```python
from build123d import *

# Parameters (mm, degrees)
SKETCH1_R           = 13.85
BOSS_EXTRUDE1_DEPTH = 12.3
SKETCH2_R           = 8.625
BOSS_EXTRUDE2_DEPTH = 1.7
SKETCH3_R           = 4.6
BOSS_EXTRUDE3_DEPTH = 8
SKETCH4_R           = 2.955
BOSS_EXTRUDE4_DEPTH = 11.75
SKETCH5_R           = 1.5
BOSS_EXTRUDE5_DEPTH = 3.42


with BuildPart() as part:
    # Sketch1 → Boss-Extrude1 (new body)
    with BuildSketch(Plane(origin=(0, 0, 0), x_dir=(1, 0, 0), z_dir=(0, 1, 0))):
        with Locations(Location((0, 0, 0), (0, 0, 270))):
            Circle(SKETCH1_R)
    extrude(amount=BOSS_EXTRUDE1_DEPTH)

    # Sketch2 → Boss-Extrude2 (add)
    with BuildSketch(Plane(origin=(0, 12.3, 0), x_dir=(1, 0, 0), z_dir=(0, 1, 0))):
        with Locations(Location((0, 0, 0), (0, 0, 270))):
            Circle(SKETCH2_R)
    extrude(amount=BOSS_EXTRUDE2_DEPTH)

    # Sketch3 → Boss-Extrude3 (add)
    with BuildSketch(Plane(origin=(0, 14, 0), x_dir=(1, 0, 0), z_dir=(0, 1, 0))):
        with Locations(Location((0, 0, 0), (0, 0, 270))):
            Circle(SKETCH3_R)
    extrude(amount=BOSS_EXTRUDE3_DEPTH)

    # Sketch4 → Boss-Extrude4 (add)
    with BuildSketch(Plane(origin=(0, 22, 0), x_dir=(1, 0, 0), z_dir=(0, 1, 0))):
        with Locations(Location((0, 0, 0), (0, 0, 270))):
            Circle(SKETCH4_R)
    extrude(amount=BOSS_EXTRUDE4_DEPTH)

    # Sketch5 → Boss-Extrude5 (add)
    with BuildSketch(Plane(origin=(0, 12.3, 0), x_dir=(1, 0, 0), z_dir=(0, 1, 0))):
        with Locations(Location((0, 9.7, 0), (0, 0, 228.961978667))):
            Circle(SKETCH5_R)
    extrude(amount=BOSS_EXTRUDE5_DEPTH)


solid = part.part
```
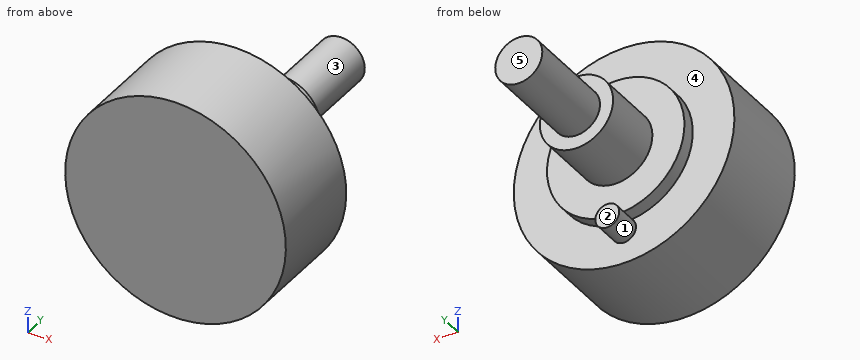
Build history of the part. All positions in model axes, mm. Face numbers are marked on the shaded views. A direction names the side the tool comes from. Give positions to 0.01 mm unless a question says otherwise; leave off trailing zeros. Order: outer loops, then holes, each group sorted by start corner. A loop starts at its lowest first (then second) coordinate and runs counter-clockwise, first axis right, second up. Notation, with made-up numbers: M -22,10 L 37,10 A11 ccw 37,25 Z; hole C -21.5,13.5 d1. An arc over 180 degrees is marked long. Return JSON: item names as keys, results as strings.
Q1. Band-saw the part on B-B (z = 0). Give the cut face in (x, y) (3 decimals), then the cut area to 3 significant figures.
Answer list:
{"outline": "M -13.85,0 L 13.85,0 L 13.85,12.3 L 8.625,12.3 L 8.625,14 L 4.6,14 L 4.6,22 L 2.955,22 L 2.955,33.75 L -2.955,33.75 L -2.955,22 L -4.6,22 L -4.6,14 L -8.625,14 L -8.625,12.3 L -13.85,12.3 Z", "area": "513 mm^2"}
Q2. Band-saw the part on A-A (x = 0). Give the cut face in (y, z) (3 decimals), then the cut area to 3 significant figures.
Answer list:
{"outline": "M 0,-13.85 L 12.3,-13.85 L 12.3,-11.2 L 15.72,-11.2 L 15.72,-8.2 L 14,-8.2 L 14,-4.6 L 22,-4.6 L 22,-2.955 L 33.75,-2.955 L 33.75,2.955 L 22,2.955 L 22,4.6 L 14,4.6 L 14,8.625 L 12.3,8.625 L 12.3,13.85 L 0,13.85 Z", "area": "523 mm^2"}
Q3. Two-plate mould, pull along Z, no slides. Class the marked faces 1, 2 and 3: pulls with the +Z half, pulls with the -Z half, needs draft (parallel to the pull), parting line crosses it, or undercut.
Answer list:
{"face 1": "undercut", "face 2": "needs draft", "face 3": "parting line crosses it"}
Q4. Flat gauge pins, fed straight in: pin 1 (10 mm diameter, centred on y = 26.5, z = 1.5, fed in from -X); pin 2 (1.5 mm diameter, centred on x = -1, y = 9, fed in from -Z); pin 3 (2.5 mm diameter, centred on x = -0.5, z = -10, fed in from +Y); pin 4 (10 mm diameter, centred on x = 0, z = 10, fed in from -Y). Where does each tip first touch, or does it go through?
Answer list:
{"pin 1": "stops at x = -4.6", "pin 2": "stops at z = -13.85", "pin 3": "stops at y = 15.72", "pin 4": "stops at y = 0"}
Q5. 3-axis set-ups, long thin cutter, end or side, ignore diameter. For the marked faces 4 and 5: which of +Z, -Z, +X, -X, +Y, -Y reach the whole face in a straight line?
Answer list:
{"face 4": "+Y", "face 5": "+Z, -Z, +X, -X, +Y"}
Q6. Band-saw the part on C-C (y = 9.5). Give the cut face in (x, z).
Answer list:
{"outline": "C 0,0 d27.7"}
Q7. Wall check: probe 1 along Y at (x, z) = (-0.25, 8.5); probe 2 along Y at (x, z) = (-12.5, -5.25); probe 3 along X at (y, z) = (12, -0.25). Give the ranges that are in metal, low to high. Write a range as from..to.
Answer list:
{"probe 1": "y = 0..14", "probe 2": "y = 0..12.3", "probe 3": "x = -13.85..13.85"}
Q8. Band-saw the part on D-D (z = -9.7). Give the cut face in (x, y).
Answer list:
{"outline": "M -9.89,0 L 9.89,0 L 9.89,12.3 L 1.5,12.3 L 1.5,15.72 L -1.5,15.72 L -1.5,12.3 L -9.89,12.3 Z"}
